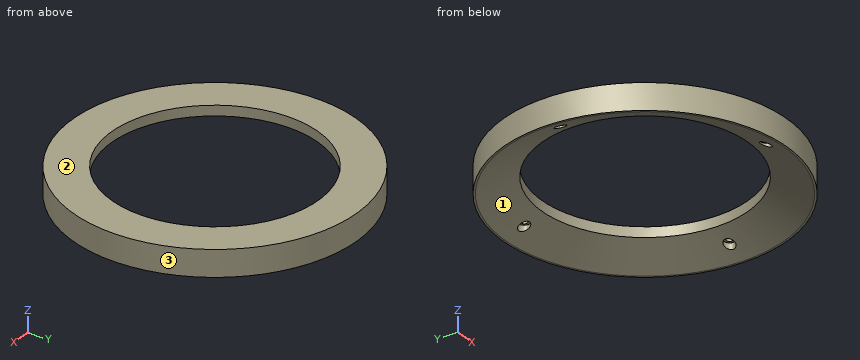
from build123d import *

# Parameters (mm, degrees)
EXPORT_R        = 70
EXPORT_R_2      = 51
PAD_DEPTH       = 13
CHAMFER_SIZE2   = 18
CHAMFER_SIZE    = 8
EXPORT001_R     = 1.5
POCKET_DEPTH    = 11
EXPORT002_R     = 2.7
POCKET001_DEPTH = 6


with BuildPart() as part:
    # Export → Pad (new body)
    with BuildSketch(Plane.XY):
        Circle(EXPORT_R)
        Circle(EXPORT_R_2, mode=Mode.SUBTRACT)
    extrude(amount=PAD_DEPTH)

    # Chamfer
    chamfer_edges = [part.edges().sort_by_distance(p)[0] for p in [
        (-51, 0, 0),
    ]]
    chamfer_side = part.faces().sort_by_distance((-51, 0, 6.5))[0]
    chamfer(chamfer_edges, length=CHAMFER_SIZE, length2=CHAMFER_SIZE2, reference=chamfer_side)

    # Export001 → Pocket (cut)
    with BuildSketch(Plane.XY):
        with Locations((0, 60)):
            Circle(EXPORT001_R)
        with Locations((60, 0)):
            Circle(EXPORT001_R)
        with Locations((0, -60)):
            Circle(EXPORT001_R)
        with Locations((-60, 0)):
            Circle(EXPORT001_R)
    extrude(amount=POCKET_DEPTH, mode=Mode.SUBTRACT)

    # Export002 → Pocket001 (cut)
    with BuildSketch(Plane.XY):
        with Locations((-60, 0)):
            Circle(EXPORT002_R)
        with Locations((0, -60)):
            Circle(EXPORT002_R)
        with Locations((0, 60)):
            Circle(EXPORT002_R)
        with Locations((60, 0)):
            Circle(EXPORT002_R)
    extrude(amount=POCKET001_DEPTH, mode=Mode.SUBTRACT)


solid = part.part
Read the model definition and answer for the solid it produces. Units are mm, in the model's axes. Face numbers are marked on the shaded views. Round coordinates to 2 decimals unless told otherwise and drop trailing zeros. One line per question, with ' | ' between items. Start each with the question number.
1. Each of these flat-tipped pins is pushed along its axis until it touches: pin 1 (2 mm diameter, centred on x = 47.5, z = 6.5, fed in from +Y); pin 2 (2.5 mm diameter, centred on x = 0.5, y = 60.5, fed in from -Z); pin 3 (2.5 mm diameter, centred on x = -1.5, y = -59, fed in from -Z). Where does it stop, or does it pass through?
2. For a pull along Y with two mould halves and no side action, classify the marked faces 1, 2 and 3 as +Y half, -Y half, draft (parallel to the pull), parting line (faces both ways), or undercut.
3. Find the intervals of material crossed by probe 1 along Y at (x, z) = (0, 8.95); probe 2 along Y at (x, z) = (0, 4.3); probe 3 along Y at (x, z) = (0, 11.2), in increasing order. Write a range as [from, to].
Filled in:
1) pin 1: y = 52.32 | pin 2: z = 6 | pin 3: z = 4.2
2) face 1: undercut | face 2: draft | face 3: parting line
3) probe 1: [-70, -61.5], [-58.5, -51], [51, 58.5], [61.5, 70] | probe 2: [-70, -62.7], [62.7, 70] | probe 3: [-70, -51], [51, 70]
